```python
from build123d import *

# Parameters (mm, degrees)
SKETCH2_R          = 1.4
CUT_EXTRUDE1_DEPTH = 6.35


with BuildPart() as part:
    # Sketch1 → Revolve1 (revolve)
    with BuildSketch(Plane.XY):
        Polygon((-29.804083682, 0), (-29.804083682, 1.534627615), (-28.915615063, 1.534627615), (-28.915615063, 2.665405858), (-27.623297071, 2.665405858), (-27.623297071, 4.765422594), (-26.694443515, 5.694276151), (-24.647883682, 5.694276151), (-24.647883682, 17.907), (-7.071083682, 17.907), (-7.071083682, 18.669), (19.979916318, 18.669), (19.979916318, 17.907), (25.440916318, 17.907), (25.440916318, 6.477), (29.809716318, 6.477), (29.809716318, 1.5875), (38.140916318, 1.5875), (38.140916318, 0), align=None)
    revolve(axis=Axis((-37.638761506, 0, 0), (1, 0, 0)))

    # Sketch2 → Cut-Extrude1 (cut)
    with BuildSketch(Plane(origin=(25.440916318, 0, 0), x_dir=(0, 0, -1), z_dir=(1, 0, 0))):
        with Locations((-12.4968, 0)):
            Circle(SKETCH2_R)
        with Locations((12.4968, 0)):
            Circle(SKETCH2_R)
    extrude(amount=-CUT_EXTRUDE1_DEPTH, mode=Mode.SUBTRACT)


solid = part.part
```
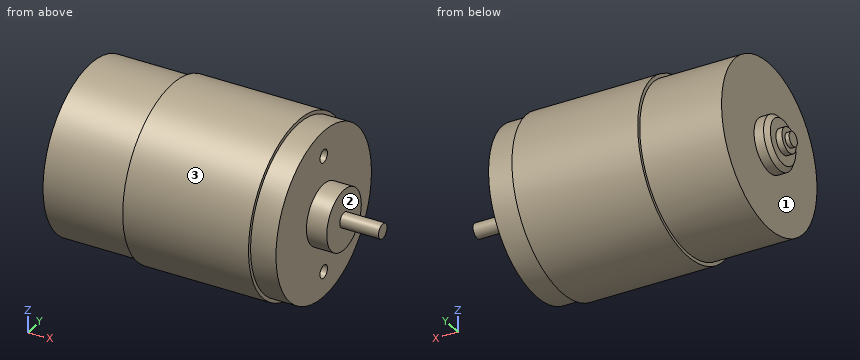
Design review of the part built by this model. Coordinates are the model's own, in mm. Face numbers are marked on the shaded views. A direction names the side the tool comes from. Round coordinates to 2 decimals unless told otherwise and drop trailing zeros. Write each loop counter-clockwise with the first axis right and the second up, starting at its lowest first coordinate (ties: lowest second). Pieces come first, ordered by that corner, then holes. Notation, with made-up numbers: (-32, 62) -> (-27, 62) arc R13 cw to (-27, 66) -> close; hole circle Ø9 at (15, -20.75). An arc over 180 degrees is marked (long way). Answer in a Markdown table with one row per item.
Q1. To check wall thickness, follow L1, parallel to X at y = 3, z = -12; L2, parallel to X at y = 2.5, z = 0; L3, parallel to Z at x = 27, y = 0. State the ranges of each line that lie inside material, in increasing order. Write a range as [from, to].
The answers:
| item | result |
|---|---|
| L1 | [-24.65, 25.44] |
| L2 | [-28.92, 29.81] |
| L3 | [-6.48, 6.48] |
Q2. Take a section at D-D, the plane x = 12.5. State the section outline as (y, z) points.
The answers:
| item | result |
|---|---|
| outline | circle Ø37.34 at (0, 0) |
Q3. Take a section at C-C, the plane y = 14.5. State the section outline as (x, z) points, then the cut area to 3 significant figures.
The answers:
| item | result |
|---|---|
| outline | (-24.65, -10.51) -> (-7.07, -10.51) -> (-7.07, -11.76) -> (19.98, -11.76) -> (19.98, -10.51) -> (25.44, -10.51) -> (25.44, 10.51) -> (19.98, 10.51) -> (19.98, 11.76) -> (-7.07, 11.76) -> (-7.07, 10.51) -> (-24.65, 10.51) -> close |
| area | 1,120 mm² |
Q4. Clearance check with flat-ended pins moving along their axes: pin 1 Ø1.5 at (x, y) = (-5, -12) entering from +Z; pin 2 Ø12 at (x, y) = (5, -12) entering from -Z; pin 3 Ø3 at (y, z) = (-0.5, -12.5) entering from +X. State where each tip first meets the part, or that it passes through.
The answers:
| item | result |
|---|---|
| pin 1 | z = 14.9 |
| pin 2 | z = -17.68 |
| pin 3 | x = 25.44 |
Q5. For the marked faces 1, 2 and 3, list the 3-axis set-ups (+Z, -Z, +X, -X, +Y, -Y) from which the entire face can be reached by the end or side of a thin tool; tool diameter is ignored.
The answers:
| item | result |
|---|---|
| face 1 | -X |
| face 2 | +X |
| face 3 | +X, -X |
Q6. Take a section at B-B, the plane x = 23. State the section outline as (y, z) points, then the cut area to 3 significant figures.
The answers:
| item | result |
|---|---|
| outline | circle Ø35.81 at (0, 0); hole circle Ø2.8 at (0, -12.5); hole circle Ø2.8 at (0, 12.5) |
| area | 995 mm² |
